Input: part model. Units: mm. Frame: model coordinates. A direction names the side the tool comes from. Coordinates: 2 decimals unless noted, no trailing zeros. Loops run counter-clockwise (first coordinate to the right, second up) from the corner with the lowest first, then second, coordinate; pieces in that order, holes last.
Item 1: Section B-B on x = 7.75. Return loops of the section in (y, z).
Item 2: Pull-direction query (Y, two-part tool) for faces 4 (the flat face through (6, 0, 30)), 5 (the flat face through (0, -32, 30)), 6 (the cylindrical face through (5.92, -73.16, 52.73)); classes: released by +Y, released by -Y, zero draft, split by the parting line, or undercut.
Item 3: Contact query for flat-ended pins moving along their axis: P1, Ø18, axis at y = -12, z = 12, coming from the +X side; P2, Ø3.5, axis at x = 14.5, z = 40.5, coming from the +Y side. Output: stop coordinate, or through.
Item 4: Reachability of faces 1 (the flat face through (16, -40, 40)), 2 (the cylindrical face through (5.916, -73.555, 7.741)), 3 (the cylindrical face through (16, -54, 30)) from +Z, -Z, +X, -X, +Y, -Y: full face, straight path, thin tool, end or side. Return the list, or none.
Item 5: Section D-D on z = 31. Return loops of the section in (x, y).
Item 6: Section A-A on z = 48. Return loops of the section in (x, y).
Item 7: Ray query, line 1 along Z through (x, y) = (7, -68); line 2 along Z through (x, y) = (9.75, -7); line 3 along X through (y, z) = (-11, 27). Return the intervals inside material, ascending.
Item 8: Section C-C on y = -68. Return loops of the section in (x, z).
```python
from build123d import *

# Parameters (mm, degrees)
F0_W     = 80
F0_H     = 60
F0_R     = 7
F1_DEPTH = 12
F2_DEPTH = 20


with BuildPart() as f1:
    # F0 (on Right) → F1 (new body)
    with BuildSketch(Plane.YZ):
        with Locations((-40, 30)):
            Rectangle(F0_W, F0_H)
        with Locations((-68, 12)):
            Circle(F0_R, mode=Mode.SUBTRACT)
        with Locations((-12, 12)):
            Circle(F0_R, mode=Mode.SUBTRACT)
        with BuildLine():
            ThreePointArc((-40, 37), (-35.050253, 34.949747), (-33, 30))
            ThreePointArc((-33, 30), (-35.050253, 25.050253), (-40, 23))
            Line((-40, 23), (-40, 16))
            ThreePointArc((-40, 16), (-54, 30), (-40, 44))
            Line((-40, 44), (-40, 37))
        make_face(mode=Mode.SUBTRACT)
        with Locations((-68, 48)):
            Circle(F0_R, mode=Mode.SUBTRACT)
        with Locations((-12, 48)):
            Circle(F0_R, mode=Mode.SUBTRACT)
    extrude(amount=F1_DEPTH)

    # F0 (on Right) → F2 (join)
    with BuildSketch(Plane.YZ):
        with BuildLine():
            ThreePointArc((-40, 23), (-47, 30), (-40, 37))
            Line((-40, 37), (-40, 44))
            ThreePointArc((-40, 44), (-54, 30), (-40, 16))
            Line((-40, 16), (-40, 23))
        make_face()
    extrude(amount=F2_DEPTH)


solid = f1.part
```
Results found:
1. outline: (-80, 0) - (0, 0) - (0, 60) - (-80, 60) - close; hole circle Ø14 at (-68, 12); hole circle Ø14 at (-68, 48); hole (-40, 23) arc R7 ccw to (-33, 30) arc R7 ccw to (-40, 37) arc R7 ccw to start; hole circle Ø14 at (-12, 12); hole circle Ø14 at (-12, 48)
2. face 4: released by +Y
2. face 5: zero draft
2. face 6: undercut
3. P1: stops at x = 12
3. P2: stops at y = -40
4. face 1: +Z, -Z, +X, +Y
4. face 2: +X, -X
4. face 3: +X, -Y
5. outline: (0, -80) - (12, -80) - (12, -53.96) - (20, -53.96) - (20, -46.93) - (0, -46.93) - close; (0, -33.07) - (12, -33.07) - (12, 0) - (0, 0) - close
6. outline: (0, -80) - (12, -80) - (12, -75) - (0, -75) - close; (0, -61) - (12, -61) - (12, -19) - (0, -19) - close; (0, -5) - (12, -5) - (12, 0) - (0, 0) - close
7. line 1: z = 0 to 5, 19 to 41, 55 to 60
7. line 2: z = 0 to 7.1, 16.9 to 43.1, 52.9 to 60
7. line 3: x = 0 to 12
8. outline: (0, 0) - (12, 0) - (12, 5) - (0, 5) - close; (0, 19) - (12, 19) - (12, 41) - (0, 41) - close; (0, 55) - (12, 55) - (12, 60) - (0, 60) - close
